Geometry: see drawing. Coordinates: mm, zero at the bounding-box minimum. Coordinates: 2 decimals unless noted, no trailing zeros. Write each loop counter-clockwise with the first axis right and the second up, starting at its lowest first coordinate (ties: lowest second). Pieces come first, ordered by that corner, then holes.
1) Section query D-D (x = 45.5). Output: boundary loops of the cut face in (y, z), then the cut area to 3 significant figures.
2) Section query A-A (z = 66). Output: boundary loops of the cut face in (x, y).
3) Line query: L1, parallel to Z at x = 54.5, y = 1.1; L2, parallel to Z at x = 34.5, y = 1.9; L3, parallel to X at y = 2.45, z = 114. Output: solid intervals per line, ascending.
4) Section query C-C (y = 0.7). State how many separate pieces and enclosed holes the cut face has, then the cut area to 3 significant figures.
5) Section query B-B (x = 144.5). Output: boundary loops of the cut face in (y, z).
6) Pin query (flat end, axial travel): pin 1 Ø3 at (x, z) = (54.5, 131.5) entering from +Y; pin 2 Ø0.8 at (y, z) = (1, 71.5) entering from +X; pin 3 Ø1.3 at (x, y) = (126, 2) entering from -Z. Return the tip coordinate at first contact, or that it passes through.
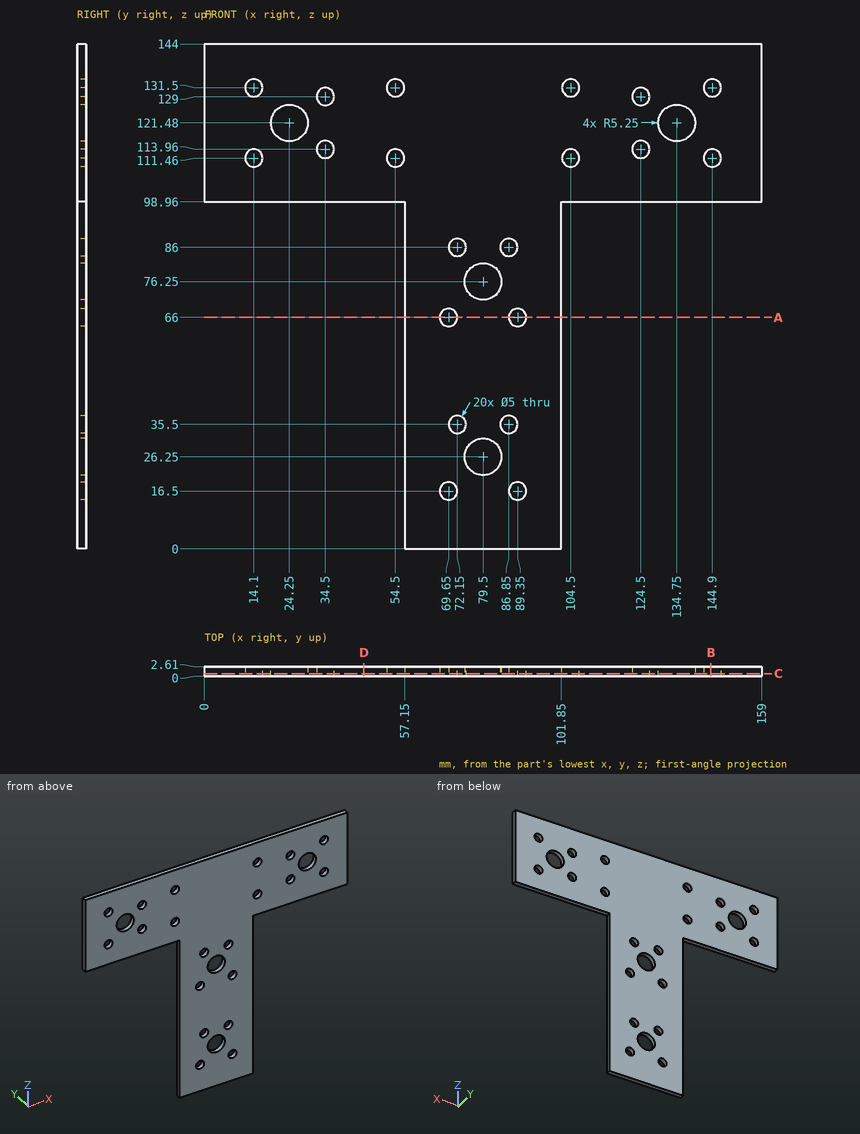
Answer:
1. outline: (0, 98.96) - (2.61, 98.96) - (2.61, 144) - (0, 144) - close
1. area: 118 mm2
2. outline: (57.15, 0) - (67.15, 0) - (67.15, 2.61) - (57.15, 2.61) - close; (72.15, 0) - (86.85, 0) - (86.85, 2.61) - (72.15, 2.61) - close; (91.85, 0) - (101.85, 0) - (101.85, 2.61) - (91.85, 2.61) - close
3. L1: z = 98.96 to 108.96, 113.96 to 129, 134 to 144
3. L2: z = 98.96 to 111.46, 116.46 to 126.5, 131.5 to 144
3. L3: x = 0 to 32, 37 to 122, 127 to 159
4. separate pieces: 1
4. enclosed holes: 24
4. area: 10,800 mm2
5. outline: (0, 98.96) - (2.61, 98.96) - (2.61, 108.99) - (0, 108.99) - close; (0, 113.93) - (2.61, 113.93) - (2.61, 129.03) - (0, 129.03) - close; (0, 133.97) - (2.61, 133.97) - (2.61, 144) - (0, 144) - close
6. pin 1: passes through
6. pin 2: stops at x = 101.85
6. pin 3: stops at z = 98.96
